from build123d import *

# Parameters (mm, degrees)
CIRPATTERN1_COUNT        = 6
FILLET1_R                = 3
BOSS_EXTRUDE1_START      = 14.8
BOSS_EXTRUDE1_DEPTH      = 3
FILLET2_R                = 3
CIRPATTERN2_COUNT        = 3
FILLET2_OF_CIRPATTERN2_R = 3


with BuildPart() as part:
    # Sketch3 → Cap (revolve)
    with BuildSketch(Plane.XY):
        Polygon((-55, 9.3), (-52.5, 9.3), (-52.5, 14.8), (-63.2, 14.8), (-63.2, 11.8), (-55, 11.8), align=None)
    revolve(axis=Axis((0, 0, 0), (0, 1, 0)))

    # Sketch12 → CSK for M3 Flat Head Machine Screw1 (revolve, cut)
    with BuildSketch(Plane(origin=(-59.2, 14.8, 0), x_dir=(0, 0, 1), z_dir=(1, 0, 0))):
        Polygon((0, 0), (0, 9.791291), (1.5, 8.89), (1.5, 1.6), (3.1, 0), align=None)
    csk_for_m3_flat_head_machine_screw1 = revolve(axis=Axis((-59.2, 21.15, 0), (0, -1, 0)), mode=Mode.SUBTRACT)

    # CirPattern1: CSK for M3 Flat Head Machine Screw1 ×6 about axis
    cirpattern1_axis = Axis((0, 0, 0), (0, 1, 0))
    for i in range(1, CIRPATTERN1_COUNT):
        add(csk_for_m3_flat_head_machine_screw1.rotate(cirpattern1_axis, i * 360 / CIRPATTERN1_COUNT), mode=Mode.SUBTRACT)

    # Fillet1
    fillet1_edges = [part.edges().sort_by_distance(p)[0] for p in [
        (52.5, 14.8, 0),
    ]]
    fillet(fillet1_edges, radius=FILLET1_R)

    # Sketch14 → Boss-Extrude1 (add)
    with BuildSketch(Plane(origin=(0, 0, 0), x_dir=(1, 0, 0), z_dir=(0, 1, 0)).offset(BOSS_EXTRUDE1_START)):
        Polygon((-63.794983, -29.903848), (-57.794983, -40.296152), (-51.485594, -36.653425), (-57.485594, -26.26112), align=None)
    boss_extrude1 = extrude(amount=-BOSS_EXTRUDE1_DEPTH)

    # Fillet2
    fillet2_edges = [part.edges().sort_by_distance(p)[0] for p in [
        (-57.794983, 13.3, 40.296152),
        (-63.794983, 13.3, 29.903848),
        (-57.485594, 13.3, 26.26112),
        (-51.485594, 13.3, 36.653425),
    ]]
    fillet(fillet2_edges, radius=FILLET2_R)

    # CirPattern2: Boss-Extrude1 ×3 about axis
    cirpattern2_axis = Axis((0, 0, 0), (0, 1, 0))
    for i in range(1, CIRPATTERN2_COUNT):
        add(boss_extrude1.rotate(cirpattern2_axis, i * 360 / CIRPATTERN2_COUNT))

    # Fillet2 of CirPattern2
    fillet2_of_cirpattern2_edges = [part.edges().sort_by_distance(p)[0] for p in [
        (63.794983, 13.3, 29.903848),
        (57.794983, 13.3, 40.296152),
        (51.485594, 13.3, 36.653425),
        (57.485594, 13.3, 26.26112),
        (-6, 13.3, -70.2),
        (6, 13.3, -70.2),
        (6, 13.3, -62.914545),
        (-6, 13.3, -62.914545),
    ]]
    fillet(fillet2_of_cirpattern2_edges, radius=FILLET2_OF_CIRPATTERN2_R)


solid = part.part
Model file for the job. Use its own axes, mm. A direction names the side the tool comes from. Round coordinates to 2 decimals unless told otherwise and drop trailing zeros. Loops run counter-clockwise (first coordinate to the right, second up) from the corner with the lowest first, then second, coordinate; pieces in that order, holes last. Notation, with made-up numbers: (68.25, -23.5) -> (115.25, -23.5) arc R35 cw to (115.25, 11.5) -> close; hole circle Ø11 at (88, -20). An arc over 180 degrees is marked (long way). Answer as CSV lines item,"result". Start each with the question number.
1) Tool access for faces 1 (the face through (11.923, 10.532, -53.692)), 2 (the face through (-6.719, 13.279, -63.636)): list every direction of +Z, -Z, +X, -X, +Y, -Y with a clear straight run to the whole face (end or side of a thin tool).
2) Slice it at C-C (y = 10.45). List the corners of the cut face in (x, z), plus the area to 3 significant figures.
3) Mould opens along X. For faces 3 (the face through (62.586, 13.279, 30.194)), 4 (the face through (30.51, 12.51, -52.46)), 5 (the face through (30.175, 12.51, 52.654)), 6 (the face through (-49, 9.3, -20)) say: +X half, -X half, draft (parallel to the pull), parting line (faces both ways), or undercut.
4) Pin check, flat tips, straight feed: P1, Ø0.8, axis at y = 14, z = -66, coming from the -X side; P2, Ø5, axis at x = -29.6, z = -51.27, coming from the +Y side; P3, Ø4, axis at x = 29.6, z = -51.27, coming from the -Y side; P4, Ø1.8, axis at x = 59.2, z = 0, coming from the +Y side. Stop position of each tip, or through.
5) Slice it at A-A (x = 0). List the corners of the cut face in (y, z).
6) Slice it at B-B (z = 0). List the corners of the cut face in (x, y), plus the area to 3 significant figures.
7) Probe line 1 along X through (y, z) = (12.5, 12); line 2 along X through (y, z) = (13.7, -13.5); line 3 along Z through (x, y) = (48, 9.9). List the from-to ranges inside material, lowest first.
Filled in:
1,face 1,"-Y"
1,face 2,"-Z, -X, +Y, -Y"
2,outline,"circle Ø110 at (0, 0); hole circle Ø105 at (0, 0)"
2,area,"844 mm2"
3,face 3,"+X half"
3,face 4,"undercut"
3,face 5,"undercut"
3,face 6,"draft"
4,P1,"stops at x = -6"
4,P2,"stops at y = 14.2"
4,P3,"stops at y = 11.8"
4,P4,"passes through"
5,outline,"(9.3, -55) -> (11.8, -55) -> (11.8, -70.2) -> (14.8, -70.2) -> (14.8, -55.5) arc R3 ccw to (11.8, -52.5) -> (9.3, -52.5) -> close; (9.3, 52.5) -> (11.8, 52.5) arc R3 ccw to (14.8, 55.5) -> (14.8, 63.2) -> (11.8, 63.2) -> (11.8, 55) -> (9.3, 55) -> close"
6,outline,"(-63.2, 11.8) -> (-60.7, 11.8) -> (-60.7, 13.2) -> (-62.3, 14.8) -> (-63.2, 14.8) -> close; (-57.7, 11.8) -> (-55, 11.8) -> (-55, 9.3) -> (-52.5, 9.3) -> (-52.5, 11.8) arc R3 ccw to (-55.5, 14.8) -> (-56.1, 14.8) -> (-57.7, 13.2) -> close; (52.5, 9.3) -> (55, 9.3) -> (55, 11.8) -> (57.7, 11.8) -> (57.7, 13.2) -> (56.1, 14.8) -> (55.5, 14.8) arc R3 ccw to (52.5, 11.8) -> close; (60.7, 11.8) -> (63.2, 11.8) -> (63.2, 14.8) -> (62.3, 14.8) -> (60.7, 13.2) -> close"
6,area,"49.7 mm2"
7,line 1,"x = -62.05 to -51.2, 51.2 to 62.05"
7,line 2,"x = -61.74 to -51.44, 51.44 to 61.74"
7,line 3,"z = -26.85 to -21.27, 21.27 to 26.85"
